Autodesk Inventor part; units mm, degrees
ref_plane "Work Plane1" through (83, 0, 0) normal (-1, 0, 0) x (0, 0, 1)
ref_plane "YZ Plane" through (0, 0, 0) normal (1, 0, 0) x (0, 1, 0)
ref_plane "XZ Plane" through (0, 0, 0) normal (0, 1, 0) x (-1, 0, 0)
sketch "Sketch1" plane through (0, 0, 0) normal (0, 0, 1) x (1, 0, 0)
  line L0 (0, 0) -> (5, 0)
  line L1 (5, 0) -> (5, -18)
  line L2 (5, -18) -> (26, -18)
  line L3 (26, -18) -> (26, 0)
  line L4 (26, 0) -> (74, 0)
  arc A0 (74, 0) -> (74, 18) centre (74, 9) ccw
  line L5 (74, 18) -> (0, 18)
  line L6 (0, 18) -> (0, 0)
  circle A1 centre (20.5, -18) radius 10.5
  dimension "d0" = 5
  dimension "d1" = 18
  dimension "d2" = 21
  dimension "d3" = 18
  dimension "d4" = 48
  dimension "d5" = 18
  dimension "d6" = 9
  dimension "d7" = 74
  dimension "d8" = 21
extrude "Extrusion1" add sketch "Sketch1" along normal blind 6
sketch "Sketch2" plane through (0, 0, 0) normal (0, 0, -1) x (-1, 0, 0)
  circle A0 centre (-74, 9) radius 4.5
  arc A1 (-26, -9.0557) -> (-10, -18) centre (-20.5, -18) ccw
  circle A2 centre (-20.5, -18) radius 4.5
  point P0 (0, 0)
  dimension "d11" = 9
  dimension "d12" = 9
extrude "Extrusion2" cut sketch "Sketch2" against normal through all
sketch "Sketch3" plane through (0, 0, 0) normal (0, 0, -1) x (-1, 0, 0)
  circle A0 centre (-7, 9) radius 1.5
  circle A1 centre (-19, 9) radius 1.5
  point P0 (0, 0)
  dimension "d16" = 3
  dimension "d17" = 3
extrude "Extrusion3" cut sketch "Sketch3" against normal through all
ref_plane "Work Plane1" through (83, 0, 0) normal (-1, 0, 0) x (0, 0, 1)
sketch "Sketch4" plane through (83, 0, 0) normal (-1, 0, 0) x (0, 0, 1)
  circle A0 centre (3, 9) radius 1.5
  point P0 (0, 0)
  dimension "d22" = 3
extrude "Extrusion4" cut sketch "Sketch4" along normal blind 18
fillet "Fillet3" radius 1 8 edges at (83, 9, 0) (50, 0, 0) (37, 18, 0) (2.5, 0, 0) (5, -9, 0) (25.6235, -27.1652, 0) (7.5, -18, 0) (26, -4.5279, 0)
sketch "Sketch5" plane through (0, 18, 6) normal (0, 1, 0) x (1, 0, 0)
  circle A0 centre (69, 2.5) radius 1.5
  circle A1 centre (58, 2.5) radius 1.5
  point P0 (0, 6)
  dimension "d26" = 3
  dimension "d27" = 3
extrude "Extrusion5" cut sketch "Sketch5" against normal blind 5
sketch "Sketch6" plane through (0, 0, 6) normal (0, 0, 1) x (1, 0, 0)
  line L0 (71, 0) -> (77, 0)
  line L1 (77, 0) -> (77, 6)
  line L2 (77, 6) -> (71, 6)
  line L3 (71, 6) -> (71, 0)
  line L4 (17.5, -18) -> (23.5, -18)
  line L5 (23.5, -18) -> (23.5, -29)
  line L6 (23.5, -29) -> (17.5, -29)
  line L7 (17.5, -29) -> (17.5, -18)
  point P0 (0, 0)
  dimension "d30" = 6
  dimension "d31" = 6
  dimension "d32" = 6
  dimension "d33" = 11
extrude "Extrusion6" cut sketch "Sketch6" against normal through all
properties part number "Hand - Digit 0-1"
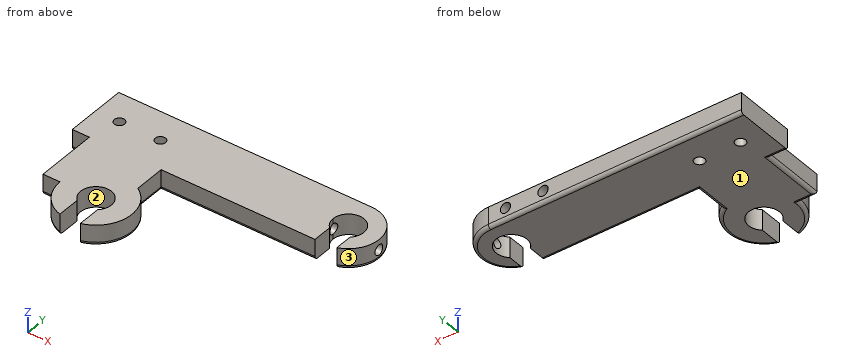
Design review of the part built by this model. Coordinates are the model's own, in mm. Face numbers are marked on the shaded views. Coordinates: 2 decimals unless noted, no trailing zeros. Order: outer loops, then holes, each group sorted by start corner. A loop starts at its lowest first (then second) coordinate and runs counter-clockwise, first axis right, second up. Notation, with made-up numbers: (24, 35) -> (43, 35) arc R31 cw to (43, 70) -> close; hole circle Ø7 at (20, -8.75). An arc over 180 degrees is marked (long way). One line per item, written item: value.
1) Clearance check with flat-ended pins moving along their axes: P1, Ø1.5, axis at x = 63.5, z = 4, coming from the -Y side; P2, Ø2.5, axis at y = -12.5, z = 4, coming from the -X side; P3, Ø1.7, axis at y = 4, z = 3.5, coming from the +X side; P4, Ø7, axis at x = 20.5, y = -18, coming from the +Z side. State where each tip first meets the part, or that it passes through.
Output values:
P1: stops at y = 0
P2: stops at x = 5
P3: stops at x = 81.99
P4: passes through
2) Draft analysis for pull direction Y (two halves, no side actions). For the marked faces 1, 2 and 3, state which applies: +Y half, -Y half, draft (parallel to the pull), parting line (faces both ways), or undercut.
Output values:
face 1: draft
face 2: undercut
face 3: parting line
3) We need section D-D, the plane x = 58. Give the boundary of the cut face in (y, z).
Output values:
outline: (0, 1) arc R1 ccw to (1, 0) -> (17, 0) arc R1 ccw to (18, 1) -> (18, 2) -> (13, 2) -> (13, 5) -> (18, 5) -> (18, 6) -> (0, 6) -> close
4) We need section C-C, the plane x = 19. Give the boundary of the cut face in (y, z), then the cut area to 3 significant figures.
Output values:
outline: (-13.76, 0) -> (7.5, 0) -> (7.5, 6) -> (-13.76, 6) -> close; (10.5, 0) -> (17, 0) arc R1 ccw to (18, 1) -> (18, 6) -> (10.5, 6) -> close
area: 172 mm2
5) We need section B-B, the plane x = 47.5. Give the boundary of the cut face in (y, z).
Output values:
outline: (0, 1) arc R1 ccw to (1, 0) -> (17, 0) arc R1 ccw to (18, 1) -> (18, 6) -> (0, 6) -> close
6) To check wall thickness, follow probe 1 along X at (y, z) = (16.9, 3.5); probe 2 along Z at (x, y) = (67.6, 9); probe 3 along Y at (x, z) = (39.5, 1.5). State the ranges of each line that lie inside material, in increasing order. Write a range as [from, to].
Output values:
probe 1: x = [0, 56.5], [59.5, 67.5], [70.5, 78.31]
probe 2: z = [0, 1.5], [4.5, 6]
probe 3: y = [0, 18]
7) We need section A-A, the plane x = 7. Give the boundary of the cut face in (y, z).
Output values:
outline: (-18, 1) arc R1 ccw to (-17, 0) -> (7.5, 0) -> (7.5, 6) -> (-18, 6) -> close; (10.5, 0) -> (17, 0) arc R1 ccw to (18, 1) -> (18, 6) -> (10.5, 6) -> close
